Geometry check sheet. Reference: drawing and pictorial views, mm from the part's lowest x, y, z. Round coordinates to 2 decimals unless told otherwise and drop trailing zeros. Order: outer loops, then holes, each group sorted by start corner. A loop starts at its lowest first (then second) coordinate and runs counter-clockwise, first axis right, second up.
Q1. Depth check by flat-ended pin: P1, Ø10, axis at y = 127, z = 42.5, coming from the -X side; P2, Ø3, axis at y = 20.5, z = 48, coming from the +X side; P3, Ø1.5, axis at y = 99, z = 76, coming from the -X side. Enter the tip coordinate at first touch or a pass-through.
Q2. Scan lines: probe 1 along X at (y, z) = (43.5, 58.5) (1 decimal); probe 2 along X at (y, z) = (76, 13); probe 3 along Z at (x, y) = (91, 20.5). Record each from-to range of solid material in increasing order.
Q3. Cross-section at C-C on x = 15.5. Record the cut outline in (y, z), then the cut area to 3 significant figures.
Q4. Cross-section at A-A on z = 43.5. Record the cut outline in (x, y) (3 decimals).
Q5. Mould release check, pull along X, two halves, no side actions. Record for the marked faces 1 and 2: +X half, -X half, draft (parallel to the pull), parting line (faces both ways), or undercut.
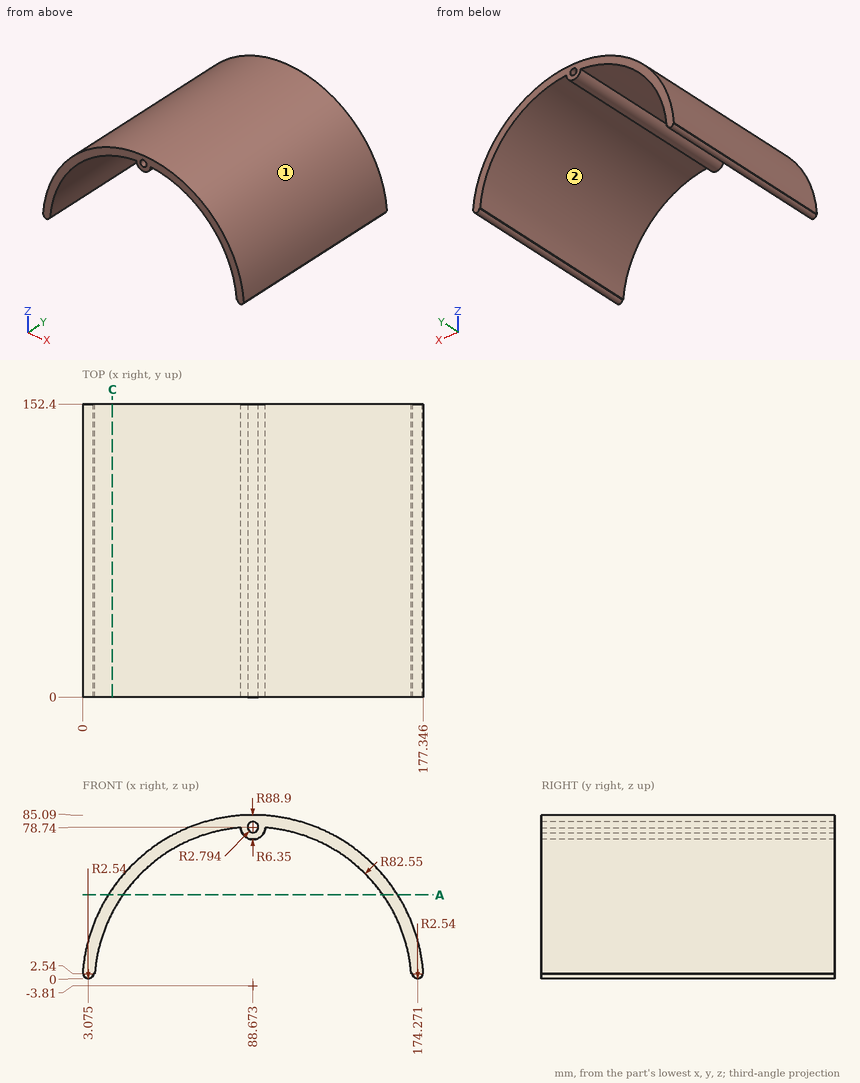
Results found:
1. P1: stops at x = 9.95
1. P2: stops at x = 161.97
1. P3: stops at x = 48.02
2. probe 1: x = 25.3 to 34.5, 142.8 to 152.1
2. probe 2: x = 1.38 to 7.85, 169.49 to 175.97
2. probe 3: z = 72.83 to 77.19, 80.29 to 85.06
3. outline: (0, 34.4) - (152.4, 34.4) - (152.4, 46.68) - (0, 46.68) - close
3. area: 1,870 mm2
4. outline: (13.407, 0) - (21.025, 0) - (21.025, 152.4) - (13.407, 152.4) - close; (156.321, 0) - (163.939, 0) - (163.939, 152.4) - (156.321, 152.4) - close
5. face 1: parting line
5. face 2: undercut
